Verification items for the finished model (mm, model axes). Face numbers are marked on the shaded views. A direction names the side the tool comes from. Give positions to 0.01 mm unless a question says otherwise; leave off trailing zeros. Loops run counter-clockwise (first coordinate to the right, second up) from the corner with the lowest first, then second, coordinate; pieces in that order, holes last. Notation, with made-up numbers: M 2,4.25 L 49,4.25 A33 ccw 49,42.25 Z; hole C -16.5,20.25 d4. An arc over 180 degrees is marked long. Answer in a Markdown table with one row per item.
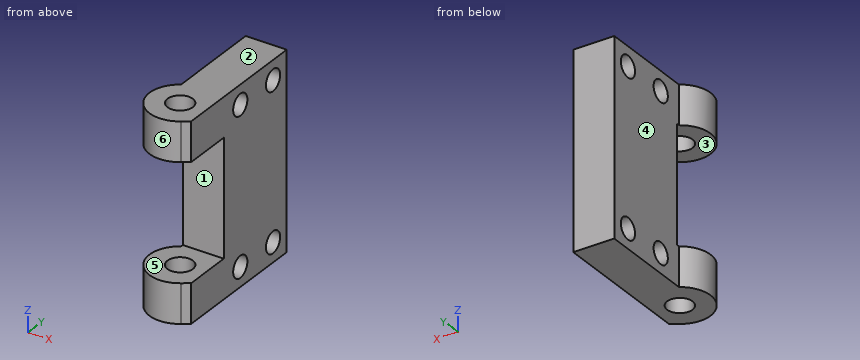
```python
from build123d import *

# Parameters (mm, degrees)
SKETCH1_R           = 3.1
BOSS_EXTRUDE1_DEPTH = 47.5
SKETCH2_W           = 28.4
SKETCH2_H           = 18.032695685
CUT_EXTRUDE1_DEPTH  = 14.5
SKETCH3_R           = 2.6
CUT_EXTRUDE2_DEPTH  = 11


with BuildPart() as part:
    # Sketch1 → Boss-Extrude1 (new body)
    with BuildSketch(Plane.XY):
        with BuildLine():
            Line((-4, 6.34428877), (-4, 30))
            Line((-4, 30), (6, 30))
            Line((6, 30), (6, -4.954564186))
            Line((6, -4.954564186), (4.301823273, -6.143640332))
            ThreePointArc((4.301823273, -6.143640332), (-6.245787992, -4.152123837), (-4, 6.34428877))
        make_face()
        Circle(SKETCH1_R, mode=Mode.SUBTRACT)
    extrude(amount=BOSS_EXTRUDE1_DEPTH)

    # Sketch2 → Cut-Extrude1 (cut, through all)
    with BuildSketch(Plane(origin=(6, 0, 0), x_dir=(0, 0, -1), z_dir=(1, 0, 0))):
        with Locations((-23.75, -2.016347843)):
            Rectangle(SKETCH2_W, SKETCH2_H)
    extrude(amount=-CUT_EXTRUDE1_DEPTH, mode=Mode.SUBTRACT)

    # Sketch3 → Cut-Extrude2 (cut, through all)
    with BuildSketch(Plane.ZY.offset(4)):
        with Locations((4.75, 25)):
            Circle(SKETCH3_R)
        with Locations((4.75, 13)):
            Circle(SKETCH3_R)
        with Locations((42.75, 25)):
            Circle(SKETCH3_R)
        with Locations((42.75, 13)):
            Circle(SKETCH3_R)
    extrude(amount=-CUT_EXTRUDE2_DEPTH, mode=Mode.SUBTRACT)


solid = part.part
```
Item 1: Sectioned sample at C-C (y = 13). Record the cut outline in (x, z).
Reported:
| item | result |
|---|---|
| outline | M -4,0 L 6,0 L 6,2.15 L -4,2.15 Z; M -4,7.35 L 6,7.35 L 6,40.15 L -4,40.15 Z; M -4,45.35 L 6,45.35 L 6,47.5 L -4,47.5 Z |
Item 2: Scan lines: L1, parallel to X at y = 0, z = 42; L2, parallel to Y at x = 0, z = 4.75; L3, parallel to Y at x = -2.5, z = 41. Record each from-to range of solid material in increasing order. Write a range as [from, to].
Reported:
| item | result |
|---|---|
| L1 | x = [-7.5, -3.1], [3.1, 6] |
| L2 | y = [-7.5, -3.1], [3.1, 10.4], [15.6, 22.4], [27.6, 30] |
| L3 | y = [-7.07, -1.83], [1.83, 11.08], [14.92, 23.08], [26.92, 30] |
Item 3: Sectioned sample at D-D (x = -6). Record the cut outline in (y, z), and give its area (3 significant figures).
Reported:
| item | result |
|---|---|
| outline | M -4.5,0 L 4.5,0 L 4.5,9.55 L -4.5,9.55 Z; M -4.5,37.95 L 4.5,37.95 L 4.5,47.5 L -4.5,47.5 Z |
| area | 172 mm^2 |
Item 4: Sectioned sample at B-B (x = 0). Record the cut outline in (y, z), and give its area (3 significant figures).
Reported:
| item | result |
|---|---|
| outline | M -7.5,0 L -3.1,0 L -3.1,9.55 L -7.5,9.55 Z; M -7.5,37.95 L -3.1,37.95 L -3.1,47.5 L -7.5,47.5 Z; M 3.1,0 L 30,0 L 30,47.5 L 3.1,47.5 L 3.1,37.95 L 7,37.95 L 7,9.55 L 3.1,9.55 Z; hole C 13,4.75 d5.2; hole C 13,42.75 d5.2; hole C 25,4.75 d5.2; hole C 25,42.75 d5.2 |
| area | 1,170 mm^2 |
Item 5: Tool access check on the marked faces 5 and 6. Record the directions out of +Z, -Z, +X, -X, +Y, -Y that give a thin tool (end or side, any length) a straight path to the whole face; none if there is none.
Reported:
| item | result |
|---|---|
| face 5 | +X, -X, -Y |
| face 6 | +Z, -Z |
Item 6: Sectioned sample at A-A (z = 42.75). Record the cut outline in (x, y).
Reported:
| item | result |
|---|---|
| outline | M -4,6.34 A7.5 ccw long 4.3,-6.14 L 6,-4.95 L 6,10.4 L -4,10.4 Z; M -4,15.6 L 6,15.6 L 6,22.4 L -4,22.4 Z; M -4,27.6 L 6,27.6 L 6,30 L -4,30 Z; hole C 0,0 d6.2 |
Item 7: Release check for a two-part mould opening along Z. For the marked faces 1, 2, 3 and 4 record: released by +Z, released by -Z, zero draft, split by the parting line, or undercut.
Reported:
| item | result |
|---|---|
| face 1 | undercut |
| face 2 | released by +Z |
| face 3 | undercut |
| face 4 | zero draft |
Item 8: Go/stop test with flat-tipped pins: pin 1 (2 mm diameter, centred on x = 3, z = 32.5, fed in from -Y); pin 2 (8.5 mm diameter, centred on y = 25, z = 42.75, fed in from -X). Record where each tip stops, or that it passes through.
Reported:
| item | result |
|---|---|
| pin 1 | stops at y = 7 |
| pin 2 | stops at x = -4 |
